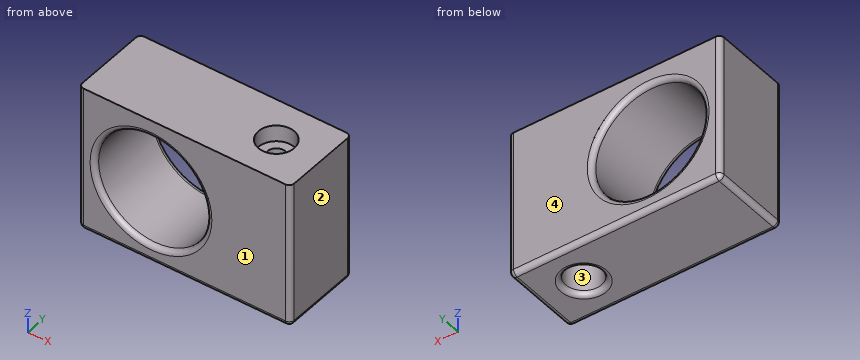
from build123d import *

# Parameters (mm, degrees)
F0_W     = 33.02
F0_H     = 12.7
F0_R     = 2.794
F1_DEPTH = 2.54
F2_W     = 33.02
F2_H     = 12.7
F2_R     = 1.397
F3_DEPTH = 2.54
F4_W     = 33.02
F4_H     = 12.7
F4_R     = 2.794
F5_DEPTH = 17.78
F6_R     = 8.73125
F7_DEPTH = 12.701
F8_R     = 0.762
F9_R     = 0.762
F10_R    = 0.762


with BuildPart() as f1:
    # F0 (on Top) → F1 (new body)
    with BuildSketch(Plane.XY):
        Rectangle(F0_W, F0_H)
        with Locations((9.561962, 0)):
            Circle(F0_R, mode=Mode.SUBTRACT)
    extrude(amount=F1_DEPTH)

    # F2 (on face) → F3 (join)
    with BuildSketch(Plane(origin=(0, 0, 0), x_dir=(1, 0, 0), z_dir=(0, 0, -1))):
        Rectangle(F2_W, F2_H)
        with Locations((9.561962, 0)):
            Circle(F2_R, mode=Mode.SUBTRACT)
    extrude(amount=F3_DEPTH)

    # F4 (on face) → F5 (join)
    with BuildSketch(Plane(origin=(0, 0, -2.54), x_dir=(1, 0, 0), z_dir=(0, 0, -1))):
        Rectangle(F4_W, F4_H)
        with Locations((9.561962, 0)):
            Circle(F4_R, mode=Mode.SUBTRACT)
    extrude(amount=F5_DEPTH)

    # F6 (on face) → F7 (cut, through all)
    with BuildSketch(Plane(origin=(0, 6.35, 0), x_dir=(-1, 0, 0), z_dir=(0, 1, 0))):
        with Locations((5.23875, -8.89)):
            Circle(F6_R)
    extrude(amount=-F7_DEPTH, mode=Mode.SUBTRACT)

    # F8
    f8_edges = [f1.edges().sort_by_distance(p)[0] for p in [
        (3.4925, -6.35, -8.89),
        (3.4925, 6.35, -8.89),
    ]]
    fillet(f8_edges, radius=F8_R)

    # F9
    f9_edges = [f1.edges().sort_by_distance(p)[0] for p in [
        (6.767962, 0, -20.32),
    ]]
    fillet(f9_edges, radius=F9_R)

    # F10
    f10_edges = [f1.edges().sort_by_distance(p)[0] for p in [
        (-16.51, 6.35, -8.89),
        (-16.51, 0, -20.32),
        (-16.51, -6.35, -8.89),
        (0, -6.35, -20.32),
        (0, 6.35, -20.32),
        (16.51, 0, -20.32),
        (16.51, 6.35, -8.89),
        (16.51, -6.35, -8.89),
    ]]
    fillet(f10_edges, radius=F10_R)


solid = f1.part
CAD build for the part. Positions are in the model's coordinates, mm. Face numbers are marked on the shaded views. Round coordinates to 2 decimals unless told otherwise and drop trailing zeros. Write each loop counter-clockwise with the first axis right and the second up, starting at its lowest first coordinate (ties: lowest second). Pieces come first, ordered by that corner, then holes.
(1) Slice it at C-C, the plane y = -4.5. Write the cut outline in (x, z).
(2) Slice it at B-B, the plane z = -8.89. Write the cut outline in (x, y), and give its area (3 significant figures).
(3) Probe line 1 along X through (y, z) = (1.75, -7); line 2 along X through (y, z) = (0, -6); line 3 along Z through (x, y) = (10.5, -1.5). List the from-to ranges inside material, lowest first.
(4) Slice it at A-A, the plane y = 0. Write the cut outline in (x, z).
(5) Drop flat-ended pins along their axis: P1, Ø1.5, axis at x = -11.5, z = -5, coming from the +Y side; P2, Ø3, axis at x = 9.56, y = 0, coming from the +Z side; P3, Ø4.5, axis at x = 9, y = 1, coming from the -Z side; P4, Ø3.5, axis at x = 9.56, y = 0, coming from the -Z side. Give the stop position or say it passes through.
(6) Mould opens along Y. For the marked faces 1, 2, 3 and 4 say: pulls with the +Y half, pulls with the -Y half, needs draft (parallel to the pull), parting line crosses it, or undercut.
From the geometry:
1. outline: (-16.51, -19.56) arc R0.76 ccw to (-15.75, -20.32) - (15.75, -20.32) arc R0.76 ccw to (16.51, -19.56) - (16.51, 2.54) - (-16.51, 2.54) - close; hole circle Ø17.46 at (-5.24, -8.89)
2. outline: (-16.51, -5.59) arc R0.76 ccw to (-15.75, -6.35) - (-14.73, -6.35) arc R0.76 ccw to (-13.97, -5.59) - (-13.97, 5.59) arc R0.76 ccw to (-14.73, 6.35) - (-15.75, 6.35) arc R0.76 ccw to (-16.51, 5.59) - close; (3.49, -5.59) arc R0.76 ccw to (4.25, -6.35) - (15.75, -6.35) arc R0.76 ccw to (16.51, -5.59) - (16.51, 5.59) arc R0.76 ccw to (15.75, 6.35) - (4.25, 6.35) arc R0.76 ccw to (3.49, 5.59) - close; hole circle Ø5.59 at (9.56, 0)
2. area: 172 mm2
3. line 1: x = -16.51 to -13.76, 3.29 to 7.38, 11.74 to 16.51
3. line 2: x = -16.51 to -13.48, 3 to 6.77, 12.36 to 16.51
3. line 3: z = -2.54 to 0
4. outline: (-16.51, -19.56) arc R0.76 ccw to (-15.75, -20.32) - (6.01, -20.32) arc R0.76 ccw to (6.77, -19.56) - (6.77, -2.54) - (8.16, -2.54) - (8.16, 0) - (6.77, 0) - (6.77, 2.54) - (-16.51, 2.54) - close; (10.96, -2.54) - (12.36, -2.54) - (12.36, -19.56) arc R0.76 ccw to (13.12, -20.32) - (15.75, -20.32) arc R0.76 ccw to (16.51, -19.56) - (16.51, 2.54) - (12.36, 2.54) - (12.36, 0) - (10.96, 0) - close; hole circle Ø17.46 at (-5.24, -8.89)
5. P1: passes through
5. P2: stops at z = 0
5. P3: stops at z = -20.3
5. P4: stops at z = -2.54
6. face 1: pulls with the -Y half
6. face 2: needs draft
6. face 3: undercut
6. face 4: pulls with the +Y half
